```python
from build123d import *

# Parameters (mm, degrees)
SKETCH1_W           = 118
SKETCH1_H           = 82
BOSS_EXTRUDE1_DEPTH = 2
CUT_EXTRUDE1_DEPTH  = 2
SKETCH3_R           = 1.5
CUT_EXTRUDE2_DEPTH  = 10


with BuildPart() as part:
    # Sketch1 → Boss-Extrude1 (new body)
    with BuildSketch(Plane(origin=(0, 0, 0), x_dir=(1, 0, 0), z_dir=(0, 1, 0))):
        Rectangle(SKETCH1_W, SKETCH1_H)
    extrude(amount=BOSS_EXTRUDE1_DEPTH)

    # Sketch2 → Cut-Extrude1 (cut)
    with BuildSketch(Plane(origin=(0, 2, 0), x_dir=(1, 0, 0), z_dir=(0, 1, 0))):
        with BuildLine():
            ThreePointArc((-44, 8), (-45.05, 6.95), (-44, 5.9))
            Line((-44, 5.9), (-44, 8))
        make_face()
        with BuildLine():
            Line((-44, 8), (-44, 5.9))
            ThreePointArc((-44, 5.9), (-43.25753788, 6.20753788), (-42.95, 6.95))
            ThreePointArc((-42.95, 6.95), (-43.25753788, 7.69246212), (-44, 8))
        make_face()
        with BuildLine():
            ThreePointArc((-44, -5.9), (-45.05, -6.95), (-44, -8))
            Line((-44, -8), (-44, -5.9))
        make_face()
        with BuildLine():
            Line((-44, -5.9), (-44, -8))
            ThreePointArc((-44, -8), (-43.25753788, -7.69246212), (-42.95, -6.95))
            ThreePointArc((-42.95, -6.95), (-43.25753788, -6.20753788), (-44, -5.9))
        make_face()
    extrude(amount=-CUT_EXTRUDE1_DEPTH, mode=Mode.SUBTRACT)

    # Sketch3 → Cut-Extrude2 (cut)
    with BuildSketch(Plane(origin=(0, 2, 0), x_dir=(1, 0, 0), z_dir=(0, 1, 0))):
        with Locations(Location((-57, 0, 0), (0, 0, 270))):
            Circle(SKETCH3_R)
        with Locations(Location((57, 0, 0), (0, 0, 90))):
            Circle(SKETCH3_R)
    extrude(amount=-CUT_EXTRUDE2_DEPTH, mode=Mode.SUBTRACT)


solid = part.part
```
Build history of the part. All positions in model axes, mm. Give positions to 0.01 mm unless a question says otherwise; leave off trailing zeros. Loops run counter-clockwise (first coordinate to the right, second up) from the corner with the lowest first, then second, coordinate; pieces in that order, holes last. Notation, with made-up numbers: (23, 88.25) -> (54, 88.25) arc R12 cw to (54, 99.25) -> close; hole circle Ø2 at (63, -13). An arc over 180 degrees is marked (long way). One line per question, with ' | ' between items.
Q1. Pull direction Z, two halves, no side cores. Call faces 1 (the cylindrical face through (-55.513, 1.014, -0.195)), 2 (the flat face through (-1, 2, -1)): pulls with the +Z half, pulls with the -Z half, needs draft (parallel to the pull), parting line crosses it, or undercut.
Filled sheet:
face 1: undercut | face 2: needs draft
Q2. Cut at B-B, the plane z = 0. Write the cut outline in (x, y).
Filled sheet:
outline: (-59, 0) -> (-58.5, 0) -> (-58.5, 2) -> (-59, 2) -> close; (-55.5, 0) -> (55.5, 0) -> (55.5, 2) -> (-55.5, 2) -> close; (58.5, 0) -> (59, 0) -> (59, 2) -> (58.5, 2) -> close
Q3. Drill centre lines: line 1 along X through (y, z) = (1.25, 0); line 2 along Z through (x, y) = (57, 0.95); line 3 along Z through (x, y) = (-44.5, 0.6). Where is each one in solid material? Low to high. Write a range as [from, to].
Filled sheet:
line 1: x = [-59, -58.5], [-55.5, 55.5], [58.5, 59] | line 2: z = [-41, -1.5], [1.5, 41] | line 3: z = [-41, -7.87], [-6.03, 6.03], [7.87, 41]
Q4. Drop flat-ended pins along their axis: pin 1 (2.5 mm diameter, centred on x = 57, z = 0, fed in from -Y); pin 2 (4 mm diameter, centred on x = -18, z = 18, fed in from -Y). Give the stop position or say it passes through.
Filled sheet:
pin 1: passes through | pin 2: stops at y = 0
Q5. Cut at A-A, the plane x = -57. Write the cut outline in (y, z), plus the area to 3 significant figures.
Filled sheet:
outline: (0, -41) -> (2, -41) -> (2, -1.5) -> (0, -1.5) -> close; (0, 1.5) -> (2, 1.5) -> (2, 41) -> (0, 41) -> close | area: 158 mm²
